Input: part model. Units: mm. Frame: model coordinates. Face numbers are marked on the shaded views. A direction names the side the tool comes from. Coordinates: 2 decimals unless noted, no trailing zeros. Order: outer loops, then holes, each group sorted by start corner. A loop starts at its lowest first (then second) coordinate and runs counter-clockwise, first axis right, second up. Notation, with made-up numbers: (67.5, 24.5) -> (102.5, 24.5) arc R30 ccw to (102.5, 58.5) -> close; hole circle Ø1 at (11.5, -11). An arc over 180 degrees is marked (long way). One line per item, written item: value. Start each with the question number.
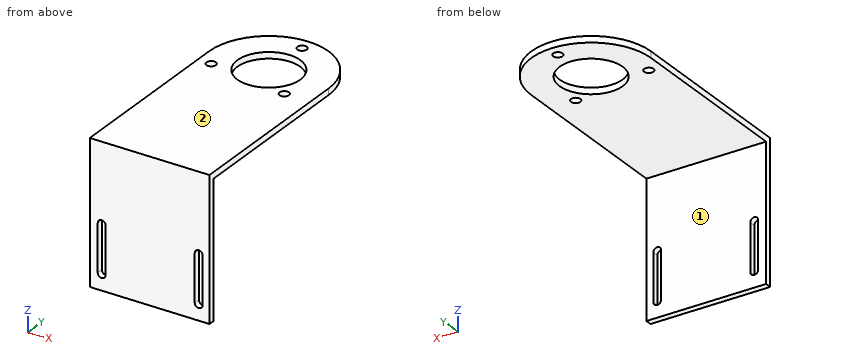
from build123d import *

# Parameters (mm, degrees)
SKETCH1_W           = 38
SKETCH1_H           = 45
BOSS_EXTRUDE1_DEPTH = 2
SKETCH3_R           = 19
SKETCH3_R_2         = 10
BOSS_EXTRUDE2_DEPTH = 2
BOSS_EXTRUDE3_DEPTH = 2
CUT_EXTRUDE1_DEPTH  = 2
SKETCH6_R           = 1.5
CUT_EXTRUDE2_DEPTH  = 2


with BuildPart() as part:
    # Sketch1 → Boss-Extrude1 (new body)
    with BuildSketch(Plane(origin=(0, 0, 0), x_dir=(1, 0, 0), z_dir=(0, 1, 0))):
        with Locations((-12.77026585, -1.948212393)):
            Rectangle(SKETCH1_W, SKETCH1_H)
    extrude(amount=BOSS_EXTRUDE1_DEPTH)



with BuildPart() as body_2:
    # Sketch3 → Boss-Extrude2 (new body)
    with BuildSketch(Plane.XY.offset(24.448212393)):
        with Locations((-12.77026585, 58)):
            Circle(SKETCH3_R)
        with Locations((-12.77026585, 58)):
            Circle(SKETCH3_R_2, mode=Mode.SUBTRACT)
    extrude(amount=-BOSS_EXTRUDE2_DEPTH)


with BuildPart() as part_1:
    add(part.part)

    add(body_2.part)  # Boss-Extrude3 merges body 2
    # Sketch3<4> → Boss-Extrude3 (add)
    with BuildSketch(Plane.XY.offset(24.448212393)):
        with BuildLine():
            Line((-31.77026585, 2), (6.22973415, 2))
            Line((6.22973415, 2), (6.22973415, 58))
            ThreePointArc((6.22973415, 58), (-12.77026585, 39), (-31.77026585, 58))
            Line((-31.77026585, 58), (-31.77026585, 2))
        make_face()
    extrude(amount=-BOSS_EXTRUDE3_DEPTH)

    # Sketch4 → Cut-Extrude1 (cut)
    with BuildSketch(Plane(origin=(0, 2, 0), x_dir=(1, 0, 0), z_dir=(0, 1, 0))):
        with BuildLine():
            Line((1.55, 0.5), (1.55, 15.5))
            ThreePointArc((1.55, 15.5), (2.8, 16.75), (4.05, 15.5))
            Line((4.05, 15.5), (4.05, 0.5))
            ThreePointArc((4.05, 0.5), (2.8, -0.75), (1.55, 0.5))
        make_face()
        with BuildLine():
            Line((-29.25, 0.5), (-29.25, 15.5))
            ThreePointArc((-29.25, 15.5), (-28, 16.75), (-26.75, 15.5))
            Line((-26.75, 15.5), (-26.75, 0.5))
            ThreePointArc((-26.75, 0.5), (-28, -0.75), (-29.25, 0.5))
        make_face()
    extrude(amount=-CUT_EXTRUDE1_DEPTH, mode=Mode.SUBTRACT)

    # Sketch6 → Cut-Extrude2 (cut)
    with BuildSketch(Plane.XY.offset(24.448212393)):
        with Locations((-12, 73)):
            Circle(SKETCH6_R)
        with Locations((-2, 49)):
            Circle(SKETCH6_R)
        with Locations((-27.5, 52.5)):
            Circle(SKETCH6_R)
    extrude(amount=-CUT_EXTRUDE2_DEPTH, mode=Mode.SUBTRACT)


solid = part_1.part
1) Access query for the marked faces 1 and 2. Directions: +Z, -Z, +X, -X, +Y, -Y. A direction counts if a zero-diameter tool reaches every point of the face in a straight line with its end or side. Return the directions, or none.
2) Section query A-A, the plane y = 55. Return the cut outline in (x, z).
3) Ray query, line 1 along Z through (x, y) = (0, 56); line 2 along Y through (x, z) = (-22, 15.5); line 3 along Y through (x, z) = (-12, 24). Return the intervals inside material, ascending. Write a range as from..to.
4) Pin query (flat end, axial travel): pin 1 Ø1.8 at (x, y) = (-27.5, 52.5) entering from -Z; pin 2 Ø10 at (x, z) = (-7, 4) entering from +Y; pin 3 Ø11.5 at (x, y) = (-22, 57.5) entering from -Z. Return the tip coordinate at first contact, or that it passes through.
5) Section query D-D, the plane z = 12. Return the cut outline in (x, y), plus the area to 3 significant figures.
6) Section query B-B, the plane x = 2.8. Return the cut outline in (y, z), plus the area to 3 significant figures.
7) Section query C-C, the plane x = -12.5. Return the cut outline in (y, z), plus the area to 3 significant figures.
Entries:
1. face 1: -Z, +X, -X, +Y
1. face 2: +Z, +X, -X, +Y, -Y
2. outline: (-31.77, 22.45) -> (-22.31, 22.45) -> (-22.31, 24.45) -> (-31.77, 24.45) -> close; (-3.23, 22.45) -> (6.23, 22.45) -> (6.23, 24.45) -> (-3.23, 24.45) -> close
3. line 1: z = 22.45..24.45
3. line 2: y = 0..2
3. line 3: y = 0..48.03, 67.97..71.5, 74.5..76.98
4. pin 1: passes through
4. pin 2: stops at y = 2
4. pin 3: stops at z = 22.45
5. outline: (-31.77, 0) -> (6.23, 0) -> (6.23, 2) -> (-31.77, 2) -> close
5. area: 76.0 mm2
6. outline: (0, -20.55) -> (2, -20.55) -> (2, -16.75) -> (0, -16.75) -> close; (0, 0.75) -> (2, 0.75) -> (2, 22.45) -> (68.89, 22.45) -> (68.89, 24.45) -> (0, 24.45) -> close
6. area: 189 mm2
7. outline: (0, -20.55) -> (2, -20.55) -> (2, 22.45) -> (48, 22.45) -> (48, 24.45) -> (0, 24.45) -> close; (68, 22.45) -> (71.59, 22.45) -> (71.59, 24.45) -> (68, 24.45) -> close; (74.41, 22.45) -> (77, 22.45) -> (77, 24.45) -> (74.41, 24.45) -> close
7. area: 194 mm2
